Can you work these out from the model? Positions are in its coordinate system, mm. Face numbers are marked on the shaded views. A direction names the side the tool comes from. Coordinates: 2 decimals unless noted, no trailing zeros. Order: outer loops, then holes, each group sorted by start corner. A loop starts at its lowest first (then second) coordinate and runs counter-clockwise, first axis right, second up.
```python
from build123d import *

# Parameters (mm, degrees)
BASPROSKE_W        = 15
BASPROSKE_H        = 12.75
TOOTHCUT_DEPTH     = 24.454743657
TEETHCUTS_COUNT    = 15
TEETHCUTS_ANGLE    = 336
BORSKE_R           = 1.5
BORE_DEPTH         = 50.0000508
SKETCH1_R          = 2.4
CUT_EXTRUDE1_DEPTH = 18


with BuildPart() as part:
    # BasProSke → Base-Revolve (revolve)
    with BuildSketch(Plane(origin=(0, 0, 0), x_dir=(1, 0, 0), z_dir=(0, 1, 0)), mode=Mode.PRIVATE) as base_revolve_sk:
        with Locations((7.5, 6.375)):
            Rectangle(BASPROSKE_W, BASPROSKE_H)
    revolve(base_revolve_sk.sketch.rotate(Axis((-10, 0, 0), (1, 0, 0)), 180), axis=Axis((-10, 0, 0), (1, 0, 0)))

    # TooCutSke → ToothCut (cut, through all)
    with BuildSketch(Plane(origin=(0, 0, 0), x_dir=(0, 0, -1), z_dir=(1, 0, 0))):
        with BuildLine():
            ThreePointArc((0.791546546, 9.340520867), (0, 9.374), (-0.791546546, 9.340520867))
            ThreePointArc((-0.791546546, 9.340520867), (-1.235070734, 11.110218102), (-2.344732916, 12.558386549))
            ThreePointArc((-2.344732916, 12.558386549), (0, 12.7754), (2.344732916, 12.558386549))
            ThreePointArc((2.344732916, 12.558386549), (1.235070734, 11.110218102), (0.791546546, 9.340520867))
        make_face()
    toothcut = extrude(amount=TOOTHCUT_DEPTH, mode=Mode.SUBTRACT)

    # TeethCuts: ToothCut ×15 about axis
    teethcuts_axis = Axis((-10, 0, 0), (1, 0, 0))
    for i in range(1, TEETHCUTS_COUNT):
        add(toothcut.rotate(teethcuts_axis, i * TEETHCUTS_ANGLE / (TEETHCUTS_COUNT - 1)), mode=Mode.SUBTRACT)

    # BorSke → Bore (cut, symmetric)
    with BuildSketch(Plane(origin=(0, 0, 0), x_dir=(0, 0, -1), z_dir=(1, 0, 0))):
        with Locations(Location((0, 0, 0), (0, 0, 180))):
            Circle(BORSKE_R)
    extrude(amount=BORE_DEPTH, both=True, mode=Mode.SUBTRACT)

    # Sketch1 → Cut-Extrude1 (cut)
    with BuildSketch(Plane(origin=(0, 0, 0), x_dir=(1, 0, 0), z_dir=(0, 1, 0))):
        with Locations(Location((7.5, 0, 0), (0, 0, 104.808618926))):
            Circle(SKETCH1_R)
    extrude(amount=CUT_EXTRUDE1_DEPTH, mode=Mode.SUBTRACT)


solid = part.part
```
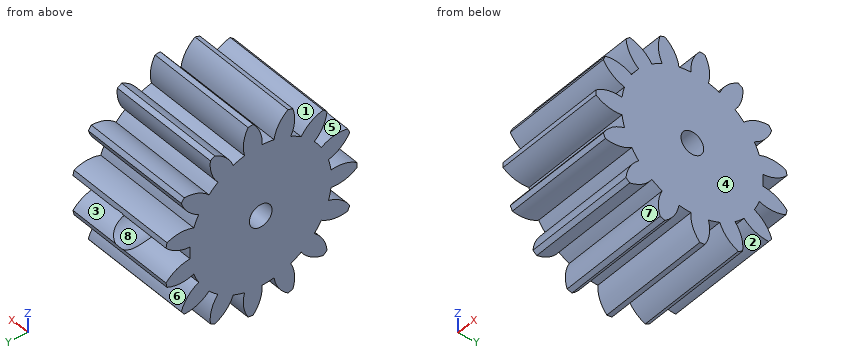
1. Please list where these lines run through material, in increasing order: probe 1 along Y at (x, z) = (10.25, 0); probe 2 along Y at (x, z) = (6, 11); probe 3 along Y at (x, z) = (7.5, 0).
Completed:
probe 1: y = -12.75 to -1.5, 1.5 to 9.37
probe 2: y = -4.48 to -2.44, 0.01 to 2.25, 5.66 to 6.45
probe 3: y = -12.75 to -1.5
2. Imagine slicing it at A-A on z = 0. Please give me the cut outline in (x, y), then the cut area to 3 significant figures.
Completed:
outline: (0, -12.75) - (15, -12.75) - (15, -1.5) - (0, -1.5) - close; (0, 1.5) - (5.1, 1.5) - (5.1, 9.37) - (0, 9.37) - close; (9.9, 1.5) - (15, 1.5) - (15, 9.37) - (9.9, 9.37) - close
area: 249 mm2
3. Thinking about a two-plate mould opening in Y: for the marked faces 6, 7 and 8, which applies, pulls with the +Y half, pulls with the -Y half, needs draft (parallel to the pull), parting line crosses it, or undercut?
Completed:
face 6: pulls with the +Y half
face 7: undercut
face 8: needs draft
4. Imagine slicing it at B-B on y = -1. Please give me the cut outline in (x, z), then the cut area to 3 significant figures.
Completed:
outline: (0, -9.32) - (15, -9.32) - (15, -1.12) - (0, -1.12) - close; (0, 1.12) - (15, 1.12) - (15, 9.32) - (0, 9.32) - close
area: 246 mm2
5. Imagine slicing it at C-C on y = 5.25. Please give me the cut outline in (x, z), then the cut area to 3 significant figures.
Completed:
outline: (0, -10.74) - (15, -10.74) - (15, 10.74) - (0, 10.74) - close; hole circle Ø4.8 at (7.5, 0)
area: 304 mm2
6. On a 3-axis mill with a long thin cutter (end or side, diameter ignored), from which of +Z, -Z, +X, -X, +Y, -Y can I reach the whole of each face in a straight line? I mean the marked faces 1, 2, 3, 4 and 5. Say none if no direction works.
Completed:
face 1: +Z, +X, -X
face 2: -Z, +X, -X
face 3: +X, -X, +Y
face 4: +Z, -Z, +X, +Y, -Y
face 5: +X, -X
7. I'm going to push flat-ended pins straight in: pin 1 (6 mm diameter, centred on x = 9.5, z = -7, fed in from -Y); pin 2 (1.5 mm diameter, centred on x = 7, y = -6, fed in from +Z); pin 3 (4 mm diameter, centred on x = 1.5, z = 7, fed in from +Y). Where does each tip first touch, or does it pass through?
Completed:
pin 1: stops at y = -11.78
pin 2: stops at z = 9.09
pin 3: stops at y = 10.51
